Geometry check sheet. Reference: the model listing, model coordinates, mm. Face numbers are marked on the shaded views. Coordinates: 2 decimals unless noted, no trailing zeros. Write each loop counter-clockwise with the first axis right and the second up, starting at its lowest first coordinate (ties: lowest second). Pieces come first, ordered by that corner, then holes.
from build123d import *

# Parameters (mm, degrees)
SKETCH_W        = 100
SKETCH_H        = 69
PAD_DEPTH       = 70
SKETCH001_W     = 90
SKETCH001_H     = 64
POCKET_DEPTH    = 67.5
SKETCH002_R     = 3.5
SKETCH002_R_2   = 1.37
PAD001_DEPTH    = 5
SKETCH003_W     = 10
SKETCH003_H     = 4
SKETCH003_W_2   = 6.5
SKETCH003_W_3   = 7
SKETCH003_H_2   = 7
POCKET001_DEPTH = 5
SKETCH004_W     = 12
SKETCH004_H     = 17
SKETCH004_W_2   = 15
SKETCH004_H_2   = 15
POCKET002_DEPTH = 5
SKETCH005_W     = 25
SKETCH005_H     = 4
POCKET003_DEPTH = 5


with BuildPart() as part:
    # Sketch → Pad (new body)
    with BuildSketch(Plane.XY):
        Rectangle(SKETCH_W, SKETCH_H)
    extrude(amount=PAD_DEPTH)

    # Sketch001 (on Face6 of Pad) → Pocket (cut)
    with BuildSketch(Plane.XY.offset(70)):
        Rectangle(SKETCH001_W, SKETCH001_H)
    extrude(amount=-POCKET_DEPTH, mode=Mode.SUBTRACT)

    # Sketch002 (on Face11 of Pocket) → Pad001 (join)
    with BuildSketch(Plane.XY.offset(2.5)):
        with Locations((-39, 24.5)):
            Circle(SKETCH002_R)
        with Locations((-39, 24.5)):
            Circle(SKETCH002_R_2, mode=Mode.SUBTRACT)
        with Locations((19, 24.5)):
            Circle(SKETCH002_R)
        with Locations((19, 24.5)):
            Circle(SKETCH002_R_2, mode=Mode.SUBTRACT)
        with Locations((-39, -24.5)):
            Circle(SKETCH002_R)
        with Locations((-39, -24.5)):
            Circle(SKETCH002_R_2, mode=Mode.SUBTRACT)
        with Locations((19, -24.5)):
            Circle(SKETCH002_R)
        with Locations((19, -24.5)):
            Circle(SKETCH002_R_2, mode=Mode.SUBTRACT)
    extrude(amount=PAD001_DEPTH)

    # Sketch003 (on Face6 of Pad001) → Pocket001 (cut)
    with BuildSketch(Plane.XZ.offset(34.5)):
        with Locations((-26.7, 14)):
            Rectangle(SKETCH003_W, SKETCH003_H)
        with Locations((-11.7, 14)):
            Rectangle(SKETCH003_W_2, SKETCH003_H)
        with Locations((1.8, 14)):
            Rectangle(SKETCH003_W_2, SKETCH003_H)
        with Locations((16.3, 15.5)):
            Rectangle(SKETCH003_W_3, SKETCH003_H_2)
    extrude(amount=-POCKET001_DEPTH, mode=Mode.SUBTRACT)

    # Sketch004 (on Face3 of Pocket001) → Pocket002 (cut)
    with BuildSketch(Plane.YZ.offset(50)):
        with Locations((-17.5, 20.5)):
            Rectangle(SKETCH004_W, SKETCH004_H)
        with Locations((0.5, 20.5)):
            Rectangle(SKETCH004_W, SKETCH004_H)
        with Locations((17.75, 19.5)):
            Rectangle(SKETCH004_W_2, SKETCH004_H_2)
    extrude(amount=-POCKET002_DEPTH, mode=Mode.SUBTRACT)

    # Sketch005 (on Face39 of Pocket002) → Pocket003 (cut)
    with BuildSketch(Plane.XY.offset(2.5)):
        with Locations((-15, 13.5)):
            Rectangle(SKETCH005_W, SKETCH005_H)
        with Locations((15, 13.5)):
            Rectangle(SKETCH005_W, SKETCH005_H)
        with Locations((-15, 4.5)):
            Rectangle(SKETCH005_W, SKETCH005_H)
        with Locations((15, 4.5)):
            Rectangle(SKETCH005_W, SKETCH005_H)
        with Locations((-15, -4.5)):
            Rectangle(SKETCH005_W, SKETCH005_H)
        with Locations((15, -4.5)):
            Rectangle(SKETCH005_W, SKETCH005_H)
        with Locations((-15, -13.5)):
            Rectangle(SKETCH005_W, SKETCH005_H)
        with Locations((15, -13.5)):
            Rectangle(SKETCH005_W, SKETCH005_H)
    extrude(amount=-POCKET003_DEPTH, mode=Mode.SUBTRACT)


solid = part.part
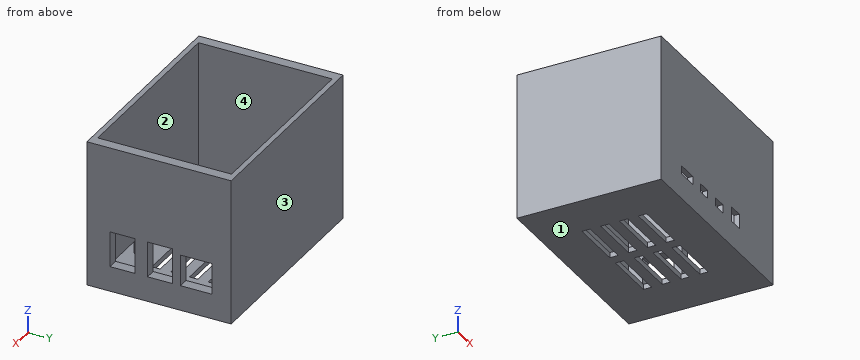
1. Thickness scan on line 1 along Y through (x, z) = (19, 5); line 2 along X through (y, z) = (-17, 62); line 3 along Y through (x, z) = (10, 46.5). Record the ranges inside material, lowest first.
Computed values:
line 1: y = -34.5 to -32, -28 to -25.87, -23.13 to -21, 21 to 23.13, 25.87 to 28, 32 to 34.5
line 2: x = -50 to -45, 45 to 50
line 3: y = -34.5 to -32, 32 to 34.5
2. Sectioned sample at D-D, the plane x = 40. Record the boundary of the cut face in (y, z).
Computed values:
outline: (-34.5, 0) - (34.5, 0) - (34.5, 70) - (32, 70) - (32, 2.5) - (-32, 2.5) - (-32, 70) - (-34.5, 70) - close
3. Gauge pin test, flat end, axial feed: pin 1 Ø2 at (x, y) = (19, 26) entering from +Z. Record the tip position at first contact, or that the pin passes through.
Computed values:
pin 1: stops at z = 7.5
4. Sectioned sample at C-C, the plane z = 48.5. Record the boundary of the cut face in (x, y), and give its area (3 significant figures).
Computed values:
outline: (-50, -34.5) - (50, -34.5) - (50, 34.5) - (-50, 34.5) - close; hole (-45, -32) - (45, -32) - (45, 32) - (-45, 32) - close
area: 1,140 mm2
5. Sectioned sample at A-A, the plane x = 9. Record the boundary of the cut face in (y, z), and give its area (3 significant figures).
Computed values:
outline: (-34.5, 0) - (-15.5, 0) - (-15.5, 2.5) - (-32, 2.5) - (-32, 70) - (-34.5, 70) - close; (-11.5, 0) - (-6.5, 0) - (-6.5, 2.5) - (-11.5, 2.5) - close; (-2.5, 0) - (2.5, 0) - (2.5, 2.5) - (-2.5, 2.5) - close; (6.5, 0) - (11.5, 0) - (11.5, 2.5) - (6.5, 2.5) - close; (15.5, 0) - (34.5, 0) - (34.5, 70) - (32, 70) - (32, 2.5) - (15.5, 2.5) - close
area: 470 mm2
6. Draft check along Y on the marked faces 1, 2, 3 and 4. Enter one of: released by +Y, released by -Y, zero draft, split by the parting line, or undercut.
Computed values:
face 1: zero draft
face 2: undercut
face 3: released by +Y
face 4: undercut
7. Sectioned sample at B-B, the plane z = 24. Record the boundary of the cut face in (x, y), and give its area (3 significant figures).
Computed values:
outline: (-50, -34.5) - (50, -34.5) - (50, -23.5) - (45, -23.5) - (45, -32) - (-45, -32) - (-45, 32) - (45, 32) - (45, 25.25) - (50, 25.25) - (50, 34.5) - (-50, 34.5) - close; (45, -11.5) - (50, -11.5) - (50, -5.5) - (45, -5.5) - close; (45, 6.5) - (50, 6.5) - (50, 10.25) - (45, 10.25) - close
area: 945 mm2
